```python
from build123d import *

# Parameters (mm, degrees)
F0_W     = 140
F0_H     = 140
F0_R     = 60
F1_DEPTH = 75
F2_R     = 65
F2_R_2   = 60
F3_DEPTH = 3.5
F4_R     = 65
F4_R_2   = 50
F5_DEPTH = 3.5
F7_DEPTH = 75.001


with BuildPart() as f1:
    # F0 (on Top) → F1 (new body)
    with BuildSketch(Plane.XY):
        Rectangle(F0_W, F0_H)
        Circle(F0_R, mode=Mode.SUBTRACT)
    extrude(amount=F1_DEPTH)

    # F2 (on face) → F3 (join)
    with BuildSketch(Plane.XY.offset(75)):
        Circle(F2_R)
        Circle(F2_R_2, mode=Mode.SUBTRACT)
    extrude(amount=F3_DEPTH)

    # F4 (on face) → F5 (cut)
    with BuildSketch(Plane(origin=(0, 0, 0), x_dir=(1, 0, 0), z_dir=(0, 0, -1))):
        Circle(F4_R)
        Circle(F4_R_2, mode=Mode.SUBTRACT)
    extrude(amount=-F5_DEPTH, mode=Mode.SUBTRACT)

    # F6 (on face) → F7 (cut, through all)
    with BuildSketch(Plane.XY.offset(75)):
        with BuildLine():
            ThreePointArc((-58.3363094479, 58.3363094479), (-56.1764068849, 60.419047572), (-53.9421968972, 62.4218663122))
            ThreePointArc((-53.9421968972, 62.4218663122), (-58.2272004968, 64.3353173023), (-62.578950135, 62.578950135))
            Line((-62.578950135, 62.578950135), (-58.3363094479, 58.3363094479))
        make_face()
        with BuildLine():
            ThreePointArc((-52.3363094479, 58.3363094479), (-52.752194688, 60.5312268377), (-53.9421968972, 62.4218663122))
            ThreePointArc((-53.9421968972, 62.4218663122), (-56.1764068849, 60.419047572), (-58.3363094479, 58.3363094479))
            Line((-58.3363094479, 58.3363094479), (-54.0936687608, 54.0936687608))
            ThreePointArc((-54.0936687608, 54.0936687608), (-52.7930322528, 56.0402088537), (-52.3363094479, 58.3363094479))
        make_face()
        with BuildLine():
            Line((-54.0936687608, 54.0936687608), (-58.3363094479, 58.3363094479))
            ThreePointArc((-58.3363094479, 58.3363094479), (-60.419047572, 56.1764068849), (-62.4218663122, 53.9421968972))
            ThreePointArc((-62.4218663122, 53.9421968972), (-58.2272004968, 52.3373015935), (-54.0936687608, 54.0936687608))
        make_face()
        with BuildLine():
            ThreePointArc((-62.4218663122, 53.9421968972), (-60.419047572, 56.1764068849), (-58.3363094479, 58.3363094479))
            Line((-58.3363094479, 58.3363094479), (-62.578950135, 62.578950135))
            ThreePointArc((-62.578950135, 62.578950135), (-64.3353173023, 58.2272004968), (-62.4218663122, 53.9421968972))
        make_face()
        with BuildLine():
            ThreePointArc((53.9421968972, 62.4218663122), (58.3363094479, 58.3363094479), (62.4218663122, 53.9421968972))
            ThreePointArc((62.4218663122, 53.9421968972), (63.836915832, 55.9397850047), (64.3363094479, 58.3363094479))
            ThreePointArc((64.3363094479, 58.3363094479), (60.5312268377, 63.9204242078), (53.9421968972, 62.4218663122))
        make_face()
        with BuildLine():
            ThreePointArc((53.9421968972, 62.4218663122), (54.0936687608, 54.0936687608), (62.4218663122, 53.9421968972))
            ThreePointArc((62.4218663122, 53.9421968972), (58.3363094479, 58.3363094479), (53.9421968972, 62.4218663122))
        make_face()
        with BuildLine():
            ThreePointArc((64.3363094479, -58.3363094479), (63.836915832, -55.9397850047), (62.4218663122, -53.9421968972))
            ThreePointArc((62.4218663122, -53.9421968972), (58.3363094479, -58.3363094479), (53.9421968972, -62.4218663122))
            ThreePointArc((53.9421968972, -62.4218663122), (60.5312268377, -63.9204242078), (64.3363094479, -58.3363094479))
        make_face()
        with BuildLine():
            ThreePointArc((53.9421968972, -62.4218663122), (58.3363094479, -58.3363094479), (62.4218663122, -53.9421968972))
            ThreePointArc((62.4218663122, -53.9421968972), (54.0936687608, -54.0936687608), (53.9421968972, -62.4218663122))
        make_face()
        with BuildLine():
            ThreePointArc((-62.4218663122, -53.9421968972), (-62.578950135, -62.578950135), (-53.9421968972, -62.4218663122))
            ThreePointArc((-53.9421968972, -62.4218663122), (-58.3363094479, -58.3363094479), (-62.4218663122, -53.9421968972))
        make_face()
        with BuildLine():
            ThreePointArc((-62.4218663122, -53.9421968972), (-58.3363094479, -58.3363094479), (-53.9421968972, -62.4218663122))
            ThreePointArc((-53.9421968972, -62.4218663122), (-52.752194688, -60.5312268377), (-52.3363094479, -58.3363094479))
            ThreePointArc((-52.3363094479, -58.3363094479), (-55.9397850047, -52.8357030638), (-62.4218663122, -53.9421968972))
        make_face()
    extrude(amount=-F7_DEPTH, mode=Mode.SUBTRACT)


solid = f1.part
```
CAD build for the part. Positions are in the model's coordinates, mm. A direction names the side the tool comes from. Give positions to 0.01 mm unless a question says otherwise; leave off trailing zeros. Order: outer loops, then holes, each group sorted by start corner. A loop starts at its lowest first (then second) coordinate and runs counter-clockwise, first axis right, second up.
(1) Tool access for faces 5 (the cylindrical face through (62, 19.52, 76.73)), 6 (the flat face through (-57.4, 31.4, 0)), 7 (the flat face through (19, 57.5, 3.5)): list every direction of +Z, -Z, +X, -X, +Y, -Y with a clear straight run to the whole face (end or side of a thin tool).
(2) Flat gauge pin, fed straight in: pin 1 (15.5 mm diameter, centred on x = 58.34, y = 58.34, fed in from +Z). Where does the tip first touch, or does it go through?
(3) Saw through at C-C, the plane y = -22.5. Give the cut face in (x, z).
(4) Saw through at A-A, the plane x = 0. Give the cut face in (y, z), then the cut area to 3 significant figures.
(5) Saw through at B-B, the plane z = 15. Give the cut face in (x, y).
(6) Drill centre lines: L1, parallel to X at y = 0, z = 29; L2, parallel to X at y = 0, z = 2.65. Where is each one in solid material? Low to high.
(7) Mould opens along X. For faces 1 (the flat face through (-70, -1, 37)), 2 (the cylindrical face through (62, -19.52, 1.73)), 3 (the flat face through (19, -57.5, 78.5)), 4 (the cylindrical face through (-59.94, 2.64, 40.48)) say: released by +X, released by -X, zero draft, split by the parting line, or undercut.
Results found:
1. face 5: +Z
1. face 6: -Z, +X, -X, +Y, -Y
1. face 7: -Z
2. pin 1: stops at z = 75
3. outline: (-70, 0) - (-60.98, 0) - (-60.98, 3.5) - (-55.62, 3.5) - (-55.62, 78.5) - (-60.98, 78.5) - (-60.98, 75) - (-70, 75) - close; (55.62, 3.5) - (60.98, 3.5) - (60.98, 0) - (70, 0) - (70, 75) - (60.98, 75) - (60.98, 78.5) - (55.62, 78.5) - close
4. outline: (-70, 0) - (-65, 0) - (-65, 3.5) - (-60, 3.5) - (-60, 78.5) - (-65, 78.5) - (-65, 75) - (-70, 75) - close; (60, 3.5) - (65, 3.5) - (65, 0) - (70, 0) - (70, 75) - (65, 75) - (65, 78.5) - (60, 78.5) - close
4. area: 1,500 mm2
5. outline: (-70, -70) - (70, -70) - (70, 70) - (-70, 70) - close; hole circle Ø12 at (-58.34, -58.34); hole circle Ø12 at (-58.34, 58.34); hole circle Ø120 at (0, 0); hole circle Ø12 at (58.34, -58.34); hole circle Ø12 at (58.34, 58.34)
6. L1: x = -70 to -60, 60 to 70
6. L2: x = -70 to -65, 65 to 70
7. face 1: released by -X
7. face 2: undercut
7. face 3: zero draft
7. face 4: undercut
